Can you work these out from the model? Positions are in its coordinate system, mm. A direction names the side the tool comes from. Round coordinates to 2 decimals unless told otherwise and drop trailing zeros. Order: outer loops, then holes, each group sorted by start corner. A loop starts at its lowest first (then second) coordinate and runs counter-clockwise, first axis right, second up. Notation, with made-up numbers: (45, 11) -> (101, 11) arc R13 ccw to (101, 34) -> close; hole circle Ø9 at (32, 61.5). An arc over 180 degrees is marked (long way). Use a Markdown table: item, result. Add a question column.
Q1. I need wall thicknesses on line 1 along Z through (x, y) = (30, -2.75); line 2 along X through (y, z) = (-2.75, 21.5); line 3 along Y through (x, z) = (28, 12). Which ranges of each line are inside material? Lowest first, please. Write a range as [from, to].
Q2. I'm going to push flat-ended pins straight in: pin 1 Ø6 at (x, z) = (28, 13) entering from +Y; pin 2 Ø6 at (x, z) = (21.5, 20.5) entering from +Y; pin 3 Ø5 at (y, z) = (11.5, 32.5) entering from +X; pin 4 Ø8 at (x, y) = (-6, 4.5) entering from +Z. Where does each tip first touch, or does it pass through?
Q3. For faces 1 (the face through (25, 0, 20)), 2 (the face through (-25, 0, 20)), 3 (the face through (9.1, 12.2, 0)), 4 (the face through (-40, -2, 20)), 5 (the face through (-15, -3, 20)), which set-ups out of +Z, -Z, +X, -X, +Y, -Y let a thin tool reach every point of the face, with its end or its side?
Q4. If we section it at B-B on z = 20: List the corners of the cut face in (x, y) for me.
Q5. We'd pull the mould along Z, two halves only. Please class faces 6 (the face through (-25, -5, 20)), 7 (the face through (30.33, -2.46, 22.48)), 8 (the face through (9.1, 12.2, 40)): +Z half, -Z half, draft (parallel to the pull), parting line (faces both ways), or undercut.
Q6. If we section it at A-A on x = 30: List the corners of the cut face in (y, z) for me, plus the area to 3 significant figures.
Q7. If we section it at D-D on z = 24: List the corners of the cut face in (x, y) for me, plus the area to 3 significant figures.
Q8. If we section it at C-C on y = -1: List the corners of the cut face in (x, z) for me, plus the area to 3 significant figures.
```python
from build123d import *

# Parameters (mm, degrees)
PAD_DEPTH    = 40
SKETCH001_R  = 2.5
POCKET_DEPTH = 5


with BuildPart() as part:
    # Sketch → Pad (new body)
    with BuildSketch(Plane.XY):
        with BuildLine():
            ThreePointArc((15, 0), (0, 15), (-15, 0))
            Line((-15, -5), (-15, 0))
            Line((-40, -5), (-15, -5))
            Line((-40, 0), (-40, -5))
            Line((-20, 0), (-40, 0))
            ThreePointArc((20, 0), (0, 20), (-20, 0))
            Line((20, 0), (40, 0))
            Line((40, 0), (40, -5))
            Line((40, -5), (15, -5))
            Line((15, -5), (15, 0))
        make_face()
    extrude(amount=PAD_DEPTH)

    # Sketch001 (on Face1 of Pad) → Pocket (cut)
    with BuildSketch(Plane(origin=(0, 0, 0), x_dir=(-1, 0, 0), z_dir=(0, 1, 0))):
        with Locations((-30, 20)):
            Circle(SKETCH001_R)
        with Locations((30, 20)):
            Circle(SKETCH001_R)
    extrude(amount=-POCKET_DEPTH, mode=Mode.SUBTRACT)


solid = part.part
```
Answer below:
| question | item | result |
|---|---|---|
| 1 | line 1 | [0, 17.5], [22.5, 40] |
| 1 | line 2 | [-40, -32], [-28, -15], [15, 28], [32, 40] |
| 1 | line 3 | [-5, 0] |
| 2 | pin 1 | y = 0 |
| 2 | pin 2 | y = 7.6 |
| 2 | pin 3 | x = 17.86 |
| 2 | pin 4 | through |
| 3 | face 1 | +Z, -Z, +X, +Y |
| 3 | face 2 | +Z, -Z, -X, +Y |
| 3 | face 3 | -Z, +X, -X, +Y, -Y |
| 3 | face 4 | +Z, -Z, -X, +Y, -Y |
| 3 | face 5 | +Z, -Z, -Y |
| 4 | outline | (-40, -5) -> (-32.5, -5) -> (-32.5, 0) -> (-40, 0) -> close; (-27.5, -5) -> (-15, -5) -> (-15, 0) arc R15 cw to (15, 0) -> (15, -5) -> (27.5, -5) -> (27.5, 0) -> (20, 0) arc R20 ccw to (-20, 0) -> (-27.5, 0) -> close; (32.5, -5) -> (40, -5) -> (40, 0) -> (32.5, 0) -> close |
| 5 | face 6 | draft |
| 5 | face 7 | undercut |
| 5 | face 8 | +Z half |
| 6 | outline | (-5, 0) -> (0, 0) -> (0, 17.5) -> (-5, 17.5) -> close; (-5, 22.5) -> (0, 22.5) -> (0, 40) -> (-5, 40) -> close |
| 6 | area | 175 mm² |
| 7 | outline | (-40, -5) -> (-15, -5) -> (-15, 0) arc R15 cw to (15, 0) -> (15, -5) -> (40, -5) -> (40, 0) -> (20, 0) arc R20 ccw to (-20, 0) -> (-40, 0) -> close |
| 7 | area | 525 mm² |
| 8 | outline | (-40, 0) -> (-15, 0) -> (-15, 40) -> (-40, 40) -> close; (15, 0) -> (40, 0) -> (40, 40) -> (15, 40) -> close; hole circle Ø5 at (-30, 20); hole circle Ø5 at (30, 20) |
| 8 | area | 1,960 mm² |
